Read the model definition and answer for the solid it produces. Units are mm, in the model's axes. Coordinates: 2 decimals unless noted, no trailing zeros. Loops run counter-clockwise (first coordinate to the right, second up) from the corner with the lowest first, then second, coordinate; pieces in that order, holes last. Notation, with made-up numbers: M 27.25,19 L 54.25,19 A9 ccw 54.25,35 Z; hole C -21,-10 d7. An arc over 180 degrees is marked long. Use one line per item in the form item = value. Start each with the question number.
1. The part is cut by section C-C (z = 2.75). Give the number of separate pieces and of enclosed holes in the cut face, plus the area to 3 significant figures.
2. The part is cut by section A-A (x = -25). Give the vertices of the cut face in (y, z), plus the area to 3 significant figures.
3. The part is cut by section D-D (x = 12.7). Give the vertices of the cut face in (y, z).
4. A flat-ended cylindrical pin translates along its axis: pin 1 (5 mm diameter, centred on x = 12.7, y = -12.7, fed in from +Z). Find the tip coordinate at first contact, or state that the pin passes through.
5. Find the intervals of material crossed by probe 1 along Y at (x, z) = (12.7, 2.85); probe 2 along Y at (x, z) = (-25, 1.7); probe 3 along X at (y, z) = (10, 2), in increasing order. Write a range as [from, to].
from build123d import *

# Parameters (mm, degrees)
SKETCH_1_W                = 60
SKETCH_1_H                = 60
EXTRUDE_1_DEPTH           = 4
HOLE_WIZARD_M3_1_D        = 2.5
HOLE_WIZARD_1_D           = 4
HOLE_WIZARD_1_CBORE_D     = 8
HOLE_WIZARD_1_CBORE_DEPTH = 3


with BuildPart() as part:
    # 草图1 → 凸台-拉伸1 (new body)
    with BuildSketch(Plane.XY):
        Rectangle(SKETCH_1_W, SKETCH_1_H)
    extrude(amount=EXTRUDE_1_DEPTH)

    # M3 螺纹孔1 (through all)
    with Locations(Plane(origin=(-25, 25, 4), x_dir=(1, 0, 0), z_dir=(0, 0, 1))):
        with Locations((0, 0), (50, 0), (50, -50), (0, -50)):
            Hole(HOLE_WIZARD_M3_1_D / 2)

    # 孔1 (through all)
    with Locations(Plane(origin=(-12.7, 12.7, 4), x_dir=(1, 0, 0), z_dir=(0, 0, 1))):
        with Locations((0, 0), (25.4, 0), (25.4, -25.4), (0, -25.4)):
            CounterBoreHole(HOLE_WIZARD_1_D / 2, HOLE_WIZARD_1_CBORE_D / 2, HOLE_WIZARD_1_CBORE_DEPTH)


solid = part.part
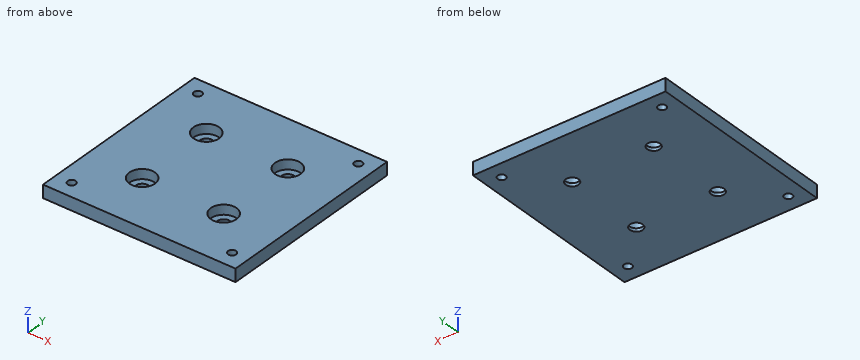
Computed values:
q1.separate_pieces = 1
q1.enclosed_holes = 8
q1.area = 3,380 mm²
q2.outline = M -30,0 L -26.25,0 L -26.25,4 L -30,4 Z; M -23.75,0 L 23.75,0 L 23.75,4 L -23.75,4 Z; M 26.25,0 L 30,0 L 30,4 L 26.25,4 Z
q2.area = 220 mm²
q3.outline = M -30,0 L -14.7,0 L -14.7,1 L -16.7,1 L -16.7,4 L -30,4 Z; M -10.7,0 L 10.7,0 L 10.7,1 L 8.7,1 L 8.7,4 L -8.7,4 L -8.7,1 L -10.7,1 Z; M 14.7,0 L 30,0 L 30,4 L 16.7,4 L 16.7,1 L 14.7,1 Z
q4.pin_1 = 1
q5.probe_1 = [-30, -16.7], [-8.7, 8.7], [16.7, 30]
q5.probe_2 = [-30, -26.25], [-23.75, 23.75], [26.25, 30]
q5.probe_3 = [-30, -15.65], [-9.75, 9.75], [15.65, 30]
